Part model, mm, in its own coordinate system. Face numbers are marked on the shaded views. A direction names the side the tool comes from. Round coordinates to 2 decimals unless told otherwise and drop trailing zeros. Order: outer loops, then holes, each group sorted by start corner. A loop starts at its lowest first (then second) coordinate and runs counter-clockwise, first axis right, second up. Notation, with made-up numbers: (-36.75, 32) - (-26.75, 32) arc R26 cw to (-26.75, 48) - close; hole circle Ø8 at (21.5, 53). An arc over 180 degrees is marked (long way). Answer as a JSON object with one key per item and string values.
Autodesk Inventor part; units mm, degrees
ref_plane "YZ Plane" through (0, 0, 0) normal (1, 0, 0) x (0, 1, 0)
ref_plane "XZ Plane" through (0, 0, 0) normal (0, 1, 0) x (-1, 0, 0)
ref_plane "XY Plane" through (0, 0, 0) normal (0, 0, 1) x (1, 0, 0)
sketch "Sketch3" plane through (0, 0, 0) normal (0, 0, 1) x (1, 0, 0)
  line L0 (0, 0) -> (103.9447, 103.9447)
  line L1 (0, 0) -> (147, 0) construction
  arc A0 (67.2085, 42.6098) -> (42.6098, 67.2085) centre (0, 0) ccw
  circle A1 centre (56.2698, 56.2698) radius 17.5
  circle A2 centre (0, 0) radius 71
  line L2 (67.2085, 42.6098) -> (63.0672, 32.6118)
  line L3 (67.2085, 42.6098) -> (78.0302, 42.6098) construction
  line L4 (42.6098, 67.2085) -> (32.6118, 63.0672)
  line L5 (42.6098, 67.2085) -> (53.4315, 67.2085) construction
  line L6 (106.7731, 99.7021) -> (12.0711, 5)
  line L7 (12.0711, 5) -> (147, 5)
  line L8 (99.7021, 106.7731) -> (-12.0711, -5)
  line L9 (-12.0711, -5) -> (147, -5)
  line L10 (103.9447, 103.9447) -> (101.1163, 106.7731)
  line L11 (103.9447, 103.9447) -> (106.7731, 101.1163)
  arc A3 (101.1163, 106.7731) -> (99.7021, 106.7731) centre (100.4092, 106.066) ccw
  arc A4 (106.7731, 99.7021) -> (106.7731, 101.1163) centre (106.066, 100.4092) ccw
  point P0 (71.6638, 64.5928)
  point P1 (64.5928, 71.6638)
  point P2 (68.6441, 68.6441)
  point P3 (70.8237, -5)
  point P4 (40.8757, 47.9468)
  point P5 (39.0352, 59.3064)
  point P6 (46.5444, 53.6155)
  point P7 (70.8237, 5)
  point P8 (47.9468, 40.8757)
  point P9 (53.6155, 46.5444)
  point P10 (59.3064, 39.0352)
  point P11 (43.8954, 43.8954)
  point P12 (50.2046, 50.2046)
  dimension "d26" = 147
  dimension "d27" = 45
  dimension "d28" = 159.1549
  dimension "d29" = 35
  dimension "d30" = 142
  dimension "d31" = 112.5
  dimension "d32" = 157.5
  dimension "d33" = 5
  dimension "d34" = 5
  dimension "d35" = 1
extrude "Extrusion2" add sketch "Sketch3" along normal blind 2 contours A2 L8 A0 L0 | L0 A0 L6 A2 | A0 L8 A1 L0 | L0 A1 L6 A0 | L6 A0 A1 A2 | A2 A1 A0 L8 | A1 L8 A3 L10 L0 | L0 L11 A4 L6 A1 | L6 A1 A0 | A0 A1 L8
sketch "Sketch4" plane through (0, 0, 2) normal (0, 0, 1) x (1, 0, 0)
  arc A0 (64.5928, 71.6638) -> (39.0352, 59.3064) centre (56.2698, 56.2698) ccw
  arc A1 (59.3064, 39.0352) -> (71.6638, 64.5928) centre (56.2698, 56.2698) ccw
  circle A2 centre (56.2698, 56.2698) radius 12.5
  line L0 (56.2698, 56.2698) -> (103.9447, 103.9447)
  line L1 (54.8556, 57.684) -> (102.5305, 105.3589)
  line L2 (57.684, 54.8556) -> (105.3589, 102.5305)
  line L3 (71.6638, 64.5928) -> (64.5928, 71.6638)
  circle A3 centre (56.2698, 56.2698) radius 7.5
  arc A4 (59.3064, 39.0352) -> (39.0352, 59.3064) centre (0, 0) ccw
  arc A5 (65.732, 33.9898) -> (33.9898, 65.732) centre (0, 0) ccw
  line L4 (103.9447, 103.9447) -> (105.3589, 102.5305)
  line L5 (106.7731, 101.1163) -> (101.1163, 106.7731)
  line L6 (102.5305, 105.3589) -> (103.9447, 103.9447)
  circle A6 centre (0, 0) radius 93.5775
  circle A7 centre (56.2698, 56.2698) radius 17.5
  point P0 (42.6098, 67.2085)
  point P1 (67.2085, 42.6098)
  point P2 (32.6118, 63.0672)
  point P3 (63.0672, 32.6118)
  point P4 (69.5425, 66.7141)
  point P5 (66.7141, 69.5425)
  point P6 (43.7753, 55.8993)
  point P7 (55.8993, 43.7753)
  point P8 (51.9915, 48.3517)
  point P9 (48.3517, 51.9915)
  point P10 (55.6314, 48.797)
  point P11 (48.797, 55.6314)
  dimension "d38" = 25
  dimension "d39" = 2
  dimension "d40" = 2
  dimension "d41" = 5
  dimension "d56" = 3
  dimension "d66" = 187.1549
  dimension "d67" = 35
extrude "Extrusion3" add sketch "Sketch4" along normal blind 20 contours L1 A7 L0 L3 | L1 L5 L0 A7 | L0 A7 L2 L3 | L0 L4 L2 A7 | A5 A3 A2 A4 | A2 L1 A3 A5 | A2 L0 A3 L1 | A5 A3 | A3 A5 | A2 L2 A3 L0 | A3 L2 A2 A5
chamfer "Chamfer6" distance 1 angle 45 9 edges at (68.1283, 68.1283, 2) (65.1086, 65.1086, 22) (84.6223, 87.4507, 22) (87.4507, 84.6223, 22) (68.1283, 68.1283, 22) (103.9447, 103.9447, 22) (84.6223, 87.4507, 2) (87.4507, 84.6223, 2) (65.1086, 65.1086, 2)
chamfer "Chamfer7" distance 2 angle 45 2 edges at (64.5928, 71.6638, 1) (71.6638, 64.5928, 1)
properties part number "HourGuard_36_wavyV2_3DPrint"
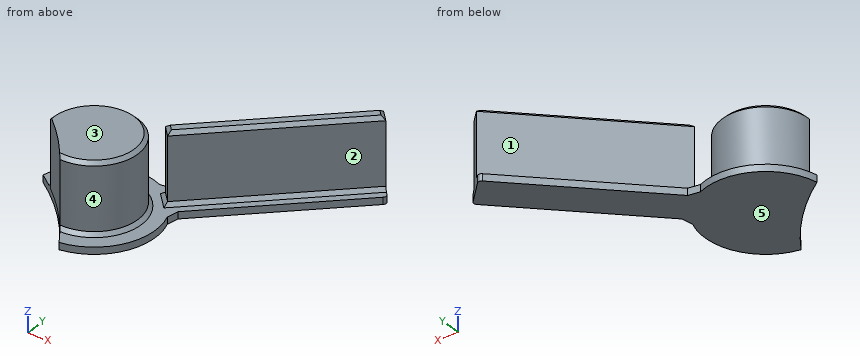
Item 1: Probe L1, parallel to Y at x = 57, z = 7.5; L2, parallel to Z at x = 92, y = 94; L3, parallel to X at y = 98, z = 11.75. List the from-to ranges inside material, lowest first. Write a range as from..to.
Taken from the geometry:
{"L1": "43.79..68.75", "L2": "0..21.59", "L3": "95.17..100.83"}
Item 2: Two-plate mould, pull along X, no slides. Class the marked faces 1, 2 and 3: pulls with the +X half, pulls with the -X half, needs draft (parallel to the pull), parting line crosses it, or undercut.
Taken from the geometry:
{"face 1": "pulls with the -X half", "face 2": "pulls with the +X half", "face 3": "needs draft"}
Item 3: Tool access for the marked faces 4 and 5: list every direction of +Z, -Z, +X, -X, +Y, -Y with a clear straight run to the whole face (end or side of a thin tool).
Taken from the geometry:
{"face 4": "+Z", "face 5": "-Z, +X, -X, +Y, -Y"}
Item 4: Cut at A-A (z = 19). Write the cut outline in (x, y), plus the area to 3 significant figures.
Taken from the geometry:
{"outline": "(43.78, 55.9) arc R71 cw to (55.9, 43.78) arc R12.5 ccw (long way) to start; (66.71, 69.54) - (69.54, 66.71) - (105.36, 102.53) - (102.53, 105.36) - close", "area": "647 mm2"}
Item 5: Cut at C-C (x = 88.5). Write the cut outline in (y, z), plus the area to 3 significant figures.
Taken from the geometry:
{"outline": "(81.43, 0) - (95.57, 0) - (95.57, 2) - (92.74, 2) - (91.33, 3) - (91.33, 21) - (89.91, 22) - (87.09, 22) - (85.67, 21) - (85.67, 3) - (84.26, 2) - (81.43, 2) - close", "area": "141 mm2"}
Item 6: Cut at B-B (y = 88). Write the cut outline in (x, z), plus the area to 3 significant figures.
Taken from the geometry:
{"outline": "(80.93, 0) - (95.07, 0) - (95.07, 2) - (92.24, 2) - (90.83, 3) - (90.83, 21) - (89.41, 22) - (86.59, 22) - (85.17, 21) - (85.17, 3) - (83.76, 2) - (80.93, 2) - close", "area": "141 mm2"}
Item 7: Drop flat-ended pins along their axis: P1, Ø1.5, axis at x = 74, y = 79.5, coming from the +Z side; P2, Ø1.5, axis at x = 94, z = 9, coming from the -Y side; P3, Ø10, axis at y = 69, z = 13, coming from the -X side. Give the stop position or say it passes through.
Taken from the geometry:
{"P1": "z = 2", "P2": "y = 90.42", "P3": "x = 46.45"}
